Could you check a few things on this drawing? It's one solid part, dimensions in mm from its lowest x, y, z. Give positions to 0.01 mm unless a question says otherwise; leave off trailing zeros. Loops run counter-clockwise (first coordinate to the right, second up) from the corner with the lowest first, then second, coordinate; pieces in that order, holes last. Notation, with made-up numbers: M 2,18 L 27,18 A28 ccw 27,39 Z; hole C -6.5,79.5 d7. An arc over 180 degrees is marked long. One line per item, written item: value. Start each with the question number.
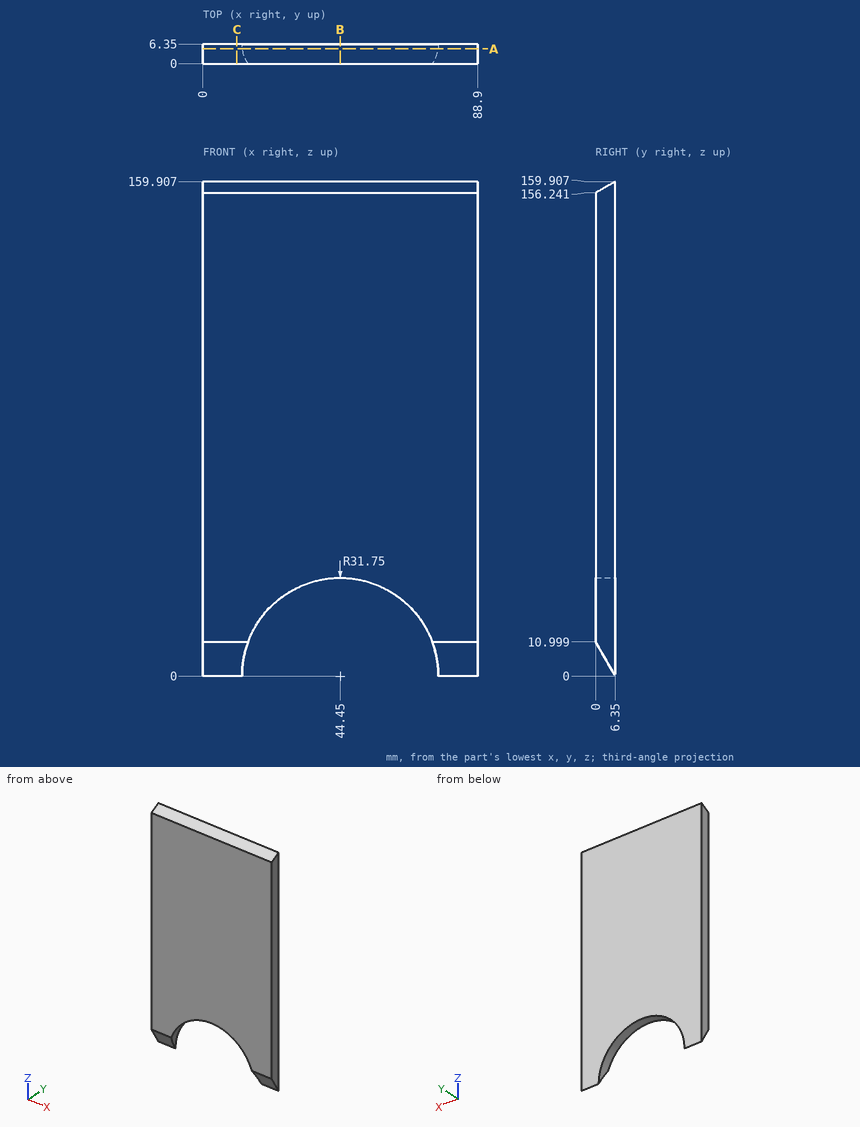
Q1. If we section it at B-B, the plane x = 44.45: Write out the boundary of the cut face in (y, z), plus the area to 3 significant figures.
Q2. If we section it at A-A, the plane y = 4.75: Write out the boundary of the cut face in (x, z).
Q3. I need wall thicknesses on line 1 along X through (y, z) = (4.75, 25.5) (1 decimal); line 2 along X through (y, z) = (4.25, 18) (1 decimal); line 3 along Z through (x, y) = (40, 5.5) (1 decimal). Which ranges of each line are inside material? Lowest first, please.
Q4. If we section it at C-C, the plane x = 11: Write out the boundary of the cut face in (y, z).
Q5. For P1, Ø2, axis at x = 66, y = 1, coming from the -Z side; P2, Ø2, axis at x = 59, y = 5, coming from the -Z side, each with a flat end and sliding along its axis, tell me the tip position at first contact or that it passes through.
Response:
1. outline: M 0,31.75 L 6.35,31.75 L 6.35,159.91 L 0,156.24 Z
1. area: 802 mm^2
2. outline: M 0,2.77 L 12.82,2.77 A31.75 cw 76.08,2.77 L 88.9,2.77 L 88.9,158.98 L 0,158.98 Z
3. line 1: 0 to 25.5, 63.4 to 88.9
3. line 2: 0 to 18.3, 70.6 to 88.9
3. line 3: 31.4 to 159.4
4. outline: M 0,11 L 6.35,0 L 6.35,159.91 L 0,156.24 Z
5. P1: z = 22.35
5. P2: z = 27.68
